Source: CAD feature listing. Evaluate the final solid. Frame: model axes, mm. Face numbers are marked on the shaded views. A direction names the side the tool comes from. Coordinates: 2 decimals unless noted, no trailing zeros. Write each loop counter-clockwise with the first axis right and the second up, starting at its lowest first coordinate (ties: lowest second). Pieces come first, ordered by that corner, then holes. Notation, with made-up numbers: (7, 57.5) - (32, 57.5) arc R19 cw to (32, 78.5) - close; hole circle Ø11 at (-21, 70.25). An arc over 180 degrees is marked (long way). One line per item, written item: value.
from build123d import *

# Parameters (mm, degrees)
F1_DEPTH = 25.4
F3_START = -50.8
F3_DEPTH = 23.6925811887
F5_START = 20.32
F4_W     = 61.8592891842
F4_H     = 58.0035075545
F5_DEPTH = 21.9097418118


with BuildPart() as f1:
    # F0 (on Front) → F1 (new body)
    with BuildSketch(Plane.XZ):
        with BuildLine():
            Line((42.2297418118, -74.4925811887), (42.2297418118, 74.4925811887))
            Line((42.2297418118, 74.4925811887), (18.1675682396, 74.4925811887))
            Line((18.1675682396, 74.4925811887), (18.1675682396, 22.7355392748))
            ThreePointArc((18.1675682396, 22.7355392748), (0.5941393293, 4.6073781801), (-18.0712514327, 21.6091079758))
            Line((-18.0712514327, 21.6091079758), (-18.0712514327, 74.4925811887))
            Line((-18.0712514327, 74.4925811887), (-42.2297418118, 74.4925811887))
            Line((-42.2297418118, 74.4925811887), (-42.2297418118, -74.4925811887))
            Line((-42.2297418118, -74.4925811887), (42.2297418118, -74.4925811887))
        make_face()
    extrude(amount=F1_DEPTH)

    # F2 (on Top) → F3 (join)
    with BuildSketch(Plane.XY.offset(F3_START)):
        with BuildLine():
            Line((42.2297418118, -91.1553874612), (42.2297418118, 0))
            Line((42.2297418118, 0), (-42.2297418118, 0))
            Line((-42.2297418118, 0), (-42.2297418118, -91.1553874612))
            ThreePointArc((-42.2297418118, -91.1553874612), (0, -133.3851292729), (42.2297418118, -91.1553874612))
        make_face()
    extrude(amount=-F3_DEPTH)

    # F4 (on Right) → F5 (cut)
    with BuildSketch(Plane.YZ.offset(F5_START)):
        with Locations((-18.2296438143, -58.8643811643)):
            Rectangle(F4_W, F4_H)
    extrude(amount=F5_DEPTH, mode=Mode.SUBTRACT)


solid = f1.part
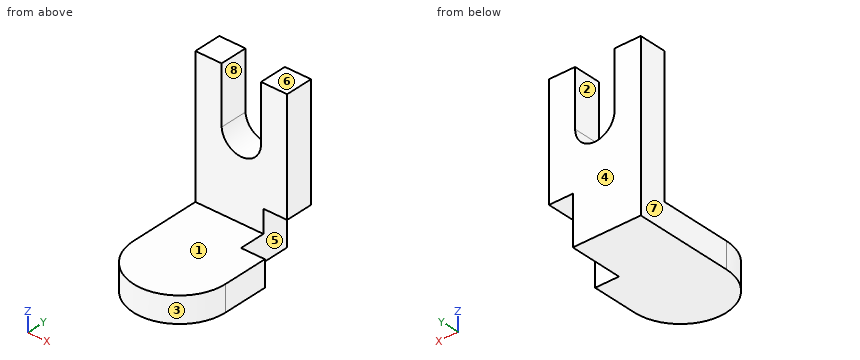
1) Draft query along X for the marked faces 6, 7 and 8. Return one class per face: released by +X, released by -X, zero draft, split by the parting line, or undercut.
Values found:
face 6: zero draft
face 7: released by -X
face 8: undercut
2) Section query B-B on z = 46.5. Output: boundary loops of the cut face in (x, y), then the cut area to 3 significant figures.
Values found:
outline: (-42.23, -25.4) - (-18.07, -25.4) - (-18.07, 0) - (-42.23, 0) - close; (18.17, -25.4) - (42.23, -25.4) - (42.23, 0) - (18.17, 0) - close
area: 1,220 mm2
3) Reachability of the marked faces 1, 2, 3, 4 and 5 from +Z, -Z, +X, -X, +Y, -Y: full face, straight path, thin tool, end or side. Return the list, or none.
Values found:
face 1: +Z, +X, -X, -Y
face 2: +Z, +Y, -Y
face 3: +Z, -Z, -Y
face 4: +Z, -Z, +X, -X, +Y
face 5: -Z, +X, +Y
4) Section query D-D on x = 0. Output: boundary loops of the cut face in (y, z).
Values found:
outline: (-133.39, -74.49) - (0, -74.49) - (0, 4.6) - (-25.4, 4.6) - (-25.4, -50.8) - (-133.39, -50.8) - close
5) Section query C-C on x = 36. Output: boundary loops of the cut face in (y, z), then the cut area to 3 significant figures.
Values found:
outline: (-113.23, -74.49) - (-49.16, -74.49) - (-49.16, -50.8) - (-113.23, -50.8) - close; (-25.4, -29.86) - (0, -29.86) - (0, 74.49) - (-25.4, 74.49) - close
area: 4,170 mm2
6) Section query A-A on y = -8.5. Output: boundary loops of the cut face in (x, z), then the cut area to 3 significant figures.
Values found:
outline: (-42.23, -74.49) - (20.32, -74.49) - (20.32, -29.86) - (42.23, -29.86) - (42.23, 74.49) - (18.17, 74.49) - (18.17, 22.74) arc R18.14 cw to (-18.07, 21.61) - (-18.07, 74.49) - (-42.23, 74.49) - close
area: 9,210 mm2
7) Material intervals for line 1 (Y direction, x = 29.5, z = 46.5); line 2 (Z direction, x = 21, y = -21); line 3 (X direction, y = -19, z = -57.5), sorted ascending.
Values found:
line 1: -25.4 to 0
line 2: -29.86 to 74.49
line 3: -42.23 to 20.32
8) Contact query for flat-ended pins moving along their axis: P1, Ø1, axis at x = -15, y = -47.5, coming from the +Z side; P2, Ø12, axis at x = -21.5, z = 49.5, coming from the +Y side; P3, Ø6.5, axis at x = 27.5, y = -16, coming from the -Z side. Output: stop coordinate, or through.
Values found:
P1: z = -50.8
P2: y = 0
P3: z = -29.86
